Can you work these out from the drawing? Everything is in mm from the part's minimum corner. A direction names the side the tool comes from. Give positions to 0.01 mm unless a question says otherwise; leave off trailing zeros. Order: outer loops, then holes, each group sorted by start corner. A loop starts at its lowest first (then second) coordinate and runs counter-clockwise, first axis right, second up. Notation, with made-up numbers: (17, 46.25) - (51, 46.25) arc R20 ccw to (51, 57.25) - close; hole circle Ø8 at (51, -3). An arc over 180 degrees is marked (long way). Answer as a JSON object with one key per item and string values.
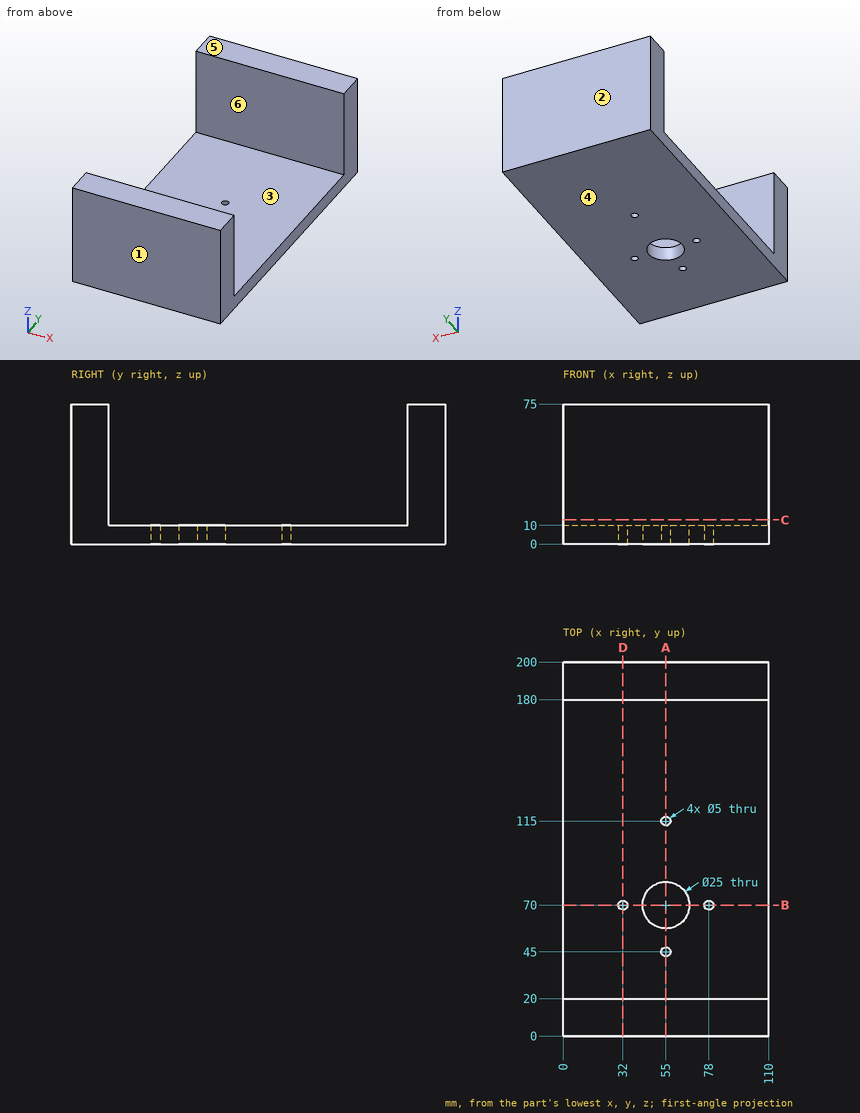
Q1. I need wall thicknesses on L1, parallel to Y at x = 55, z = 5; L2, parallel to X at y = 70, z = 6; L3, parallel to Y at x = 16.5, z = 32.5. Which ranges of each line are inside material? Lowest first, please.
Recorded:
{"L1": "y = 0 to 42.5, 47.5 to 57.5, 82.5 to 112.5, 117.5 to 200", "L2": "x = 0 to 29.5, 34.5 to 42.5, 67.5 to 75.5, 80.5 to 110", "L3": "y = 0 to 20, 180 to 200"}
Q2. If we section it at A-A, the plane x = 55: Please give me the cut outline in (y, z), then the cut area to 3 significant figures.
Recorded:
{"outline": "(0, 0) - (42.5, 0) - (42.5, 10) - (20, 10) - (20, 75) - (0, 75) - close; (47.5, 0) - (57.5, 0) - (57.5, 10) - (47.5, 10) - close; (82.5, 0) - (112.5, 0) - (112.5, 10) - (82.5, 10) - close; (117.5, 0) - (200, 0) - (200, 75) - (180, 75) - (180, 10) - (117.5, 10) - close", "area": "4,250 mm^2"}
Q3. Which directions (+Z, -Z, +X, -X, +Y, -Y) give clear straight access to the entire face, cutting with the end or side of a thin tool? Please do the marked faces 5 and 6.
Recorded:
{"face 5": "+Z, +X, -X, +Y, -Y", "face 6": "+Z, +X, -X"}
Q4. If we section it at C-C, the plane z = 13: Please give me the cut outline in (x, y), then the cut area to 3 significant figures.
Recorded:
{"outline": "(0, 0) - (110, 0) - (110, 20) - (0, 20) - close; (0, 180) - (110, 180) - (110, 200) - (0, 200) - close", "area": "4,400 mm^2"}
Q5. If we section it at B-B, the plane y = 70: Please give me the cut outline in (x, z).
Recorded:
{"outline": "(0, 0) - (29.5, 0) - (29.5, 10) - (0, 10) - close; (34.5, 0) - (42.5, 0) - (42.5, 10) - (34.5, 10) - close; (67.5, 0) - (75.5, 0) - (75.5, 10) - (67.5, 10) - close; (80.5, 0) - (110, 0) - (110, 10) - (80.5, 10) - close"}
Q6. We'd pull the mould along Y, two halves only. Please class the marked faces 1, 2, 3 and 4: released by +Y, released by -Y, zero draft, split by the parting line, or undercut.
Recorded:
{"face 1": "released by -Y", "face 2": "released by +Y", "face 3": "undercut", "face 4": "zero draft"}
Q7. If we section it at D-D, the plane x = 32: Please give me the cut outline in (y, z), then the cut area to 3 significant figures.
Recorded:
{"outline": "(0, 0) - (67.5, 0) - (67.5, 10) - (20, 10) - (20, 75) - (0, 75) - close; (72.5, 0) - (200, 0) - (200, 75) - (180, 75) - (180, 10) - (72.5, 10) - close", "area": "4,550 mm^2"}
Q8. I'm going to push a flat-ended pin straight in: pin 1 Ø1 at (x, y) = (89.5, 22) entering from +Z. Where does the tip first touch, or does it pass through?
Recorded:
{"pin 1": "stops at z = 10"}
